Here's the drawing with two shaded views (mm, measured from the low corner). I have some questions. A direction names the side the tool comes from. Round coordinates to 2 decimals unless told otherwise and drop trailing zeros. Order: outer loops, then holes, each group sorted by start corner. A loop starts at its lowest first (then second) coordinate and runs counter-clockwise, first axis right, second up.
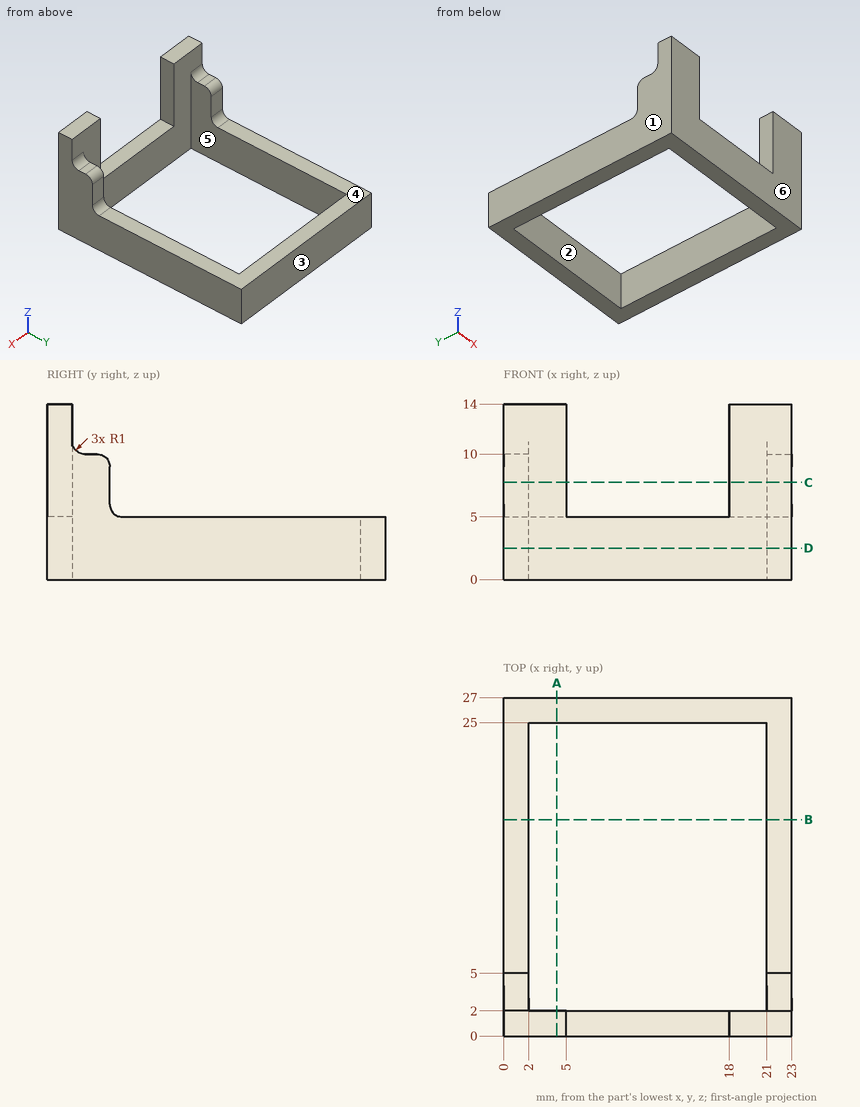
Q1. For P1, Ø1.6, axis at x = 1, z = 8, coming from the +Y side; P2, Ø1.6, axis at y = 0.5, z = 8.5, coming from the -X side; P3, Ø1.1, axis at x = 22, y = 3.5, coming from the +Z side; P4, Ø1, axis at x = 11.5, y = 1.5, coming from the +Z side, each with a flat end and sliding along its axis, tell me the tip position at first contact or that it passes through.
Q2. Imagine slicing it at C-C, the plane z = 7.75. Please give me the cut outline in (x, y).
Q3. Imagine slicing it at D-D, the plane z = 2.5. Please give me the cut outline in (x, y), then the cut area to 3 significant figures.
Q4. Imagine slicing it at B-B, the plane y = 17.25. Please give me the cut outline in (x, z), then the cut area to 3 significant figures.
Q5. Imagine slicing it at A-A, the plane x = 4.25. Please give me the cut outline in (y, z).
Q6. We'd pull the mould along Y, two halves only. Please class the marked faces 1, 2 and 3: released by +Y, released by -Y, zero draft, split by the parting line, or undercut.
Q7. I need wall thicknesses on L1, parallel to Y at x = 16, z = 3.5; L2, parallel to X at y = 20.5, z = 3; L3, parallel to Y at x = 21.25, z = 12.75. Which ranges of each line are inside material? Lowest first, please.
Q8. For the marked faces 4, 5 and 6, which set-ups out of +Z, -Z, +X, -X, +Y, -Y let a thin tool reach every point of the face, with its end or its side?
Filled in:
1. P1: stops at y = 5
1. P2: stops at x = 0
1. P3: stops at z = 10
1. P4: stops at z = 5
2. outline: (0, 0) - (5, 0) - (5, 2) - (2, 2) - (2, 5) - (0, 5) - close; (18, 0) - (23, 0) - (23, 5) - (21, 5) - (21, 2) - (18, 2) - close
3. outline: (0, 0) - (23, 0) - (23, 27) - (0, 27) - close; hole (2, 2) - (21, 2) - (21, 25) - (2, 25) - close
3. area: 184 mm2
4. outline: (0, 0) - (2, 0) - (2, 5) - (0, 5) - close; (21, 0) - (23, 0) - (23, 5) - (21, 5) - close
4. area: 20.0 mm2
5. outline: (0, 0) - (2, 0) - (2, 14) - (0, 14) - close; (25, 0) - (27, 0) - (27, 5) - (25, 5) - close
6. face 1: zero draft
6. face 2: undercut
6. face 3: released by +Y
7. L1: y = 0 to 2, 25 to 27
7. L2: x = 0 to 2, 21 to 23
7. L3: y = 0 to 2
8. face 4: +Z, +X, -X, +Y
8. face 5: +Z, -Z
8. face 6: +Z, -Z, +X, -X, -Y
